The model under review builds one solid part; all positions refer to its coordinate system, in mm. Coordinates: 2 decimals unless noted, no trailing zeros. Loops run counter-clockwise (first coordinate to the right, second up) from the corner with the lowest first, then second, coordinate; pieces in that order, holes last. Notation, with made-up numbers: M -3,-35.5 L 24,-35.5 A10 cw 24,-29.5 Z; hole C -21,66.5 d2. An arc over 180 degrees is marked long. Return JSON: item names as keys, results as strings.
```python
from build123d import *

# Parameters (mm, degrees)
SKETCH1_R           = 12
SKETCH1_R_2         = 8
BOSS_EXTRUDE1_DEPTH = 10
CHAMFER1_SIZE       = 1
SKETCH2_R           = 2
CUT_EXTRUDE1_DEPTH  = 27


with BuildPart() as part:
    # Sketch1 → Boss-Extrude1 (new body)
    with BuildSketch(Plane.XY):
        Circle(SKETCH1_R)
        Circle(SKETCH1_R_2, mode=Mode.SUBTRACT)
    extrude(amount=BOSS_EXTRUDE1_DEPTH)

    # Chamfer1
    chamfer1_edges = [part.edges().sort_by_distance(p)[0] for p in [
        (-12, 0, 10),
    ]]
    chamfer(chamfer1_edges, length=CHAMFER1_SIZE)

    # Sketch2 → Cut-Extrude1 (cut, symmetric)
    with BuildSketch(Plane(origin=(0, 0, 0), x_dir=(1, 0, 0), z_dir=(0, 1, 0))):
        with Locations(Location((0, -4.2, 0), (0, 0, 270))):
            Circle(SKETCH2_R)
    extrude(amount=CUT_EXTRUDE1_DEPTH, both=True, mode=Mode.SUBTRACT)


solid = part.part
```
1. Add section B-B on y = 0. Give the boundary of the cut face in (x, z), plus the area to 3 significant figures.
Check values:
{"outline": "M -12,0 L -8,0 L -8,10 L -11,10 L -12,9 Z; M 8,0 L 12,0 L 12,9 L 11,10 L 8,10 Z", "area": "79.0 mm²"}
2. Add section A-A on x = 0. Give the boundary of the cut face in (y, z).
Check values:
{"outline": "M -12,0 L -8,0 L -8,2.2 L -12,2.2 Z; M -12,6.2 L -8,6.2 L -8,10 L -11,10 L -12,9 Z; M 8,0 L 12,0 L 12,2.2 L 8,2.2 Z; M 8,6.2 L 12,6.2 L 12,9 L 11,10 L 8,10 Z"}
3. To check wall thickness, follow line 1 (Z direction, x = 0, y = -9.2); line 2 (X direction, y = 9.15, z = 4.2); line 3 (Y direction, x = 6.5, z = 7.5). State the ranges of each line that lie inside material, in increasing order.
Check values:
{"line 1": "0 to 2.2, 6.2 to 10", "line 2": "-7.76 to -2, 2 to 7.76", "line 3": "-10.09 to -4.66, 4.66 to 10.09"}
4. Add section D-D on z = 3.5. Give the boundary of the cut face in (x, y), plus the area to 3 significant figures.
Check values:
{"outline": "M -1.87,-11.85 L -1.87,-7.78 A8 cw -1.87,7.78 L -1.87,11.85 A12 ccw Z; M 1.87,-11.85 A12 ccw 1.87,11.85 L 1.87,7.78 A8 cw 1.87,-7.78 Z", "area": "221 mm²"}
5. The part is to be moulded in two halves that separate along Z. For faces 1 (the face through (0.088, -9.845, 2.202)), 2 (the face through (-2, -8, 10)), 3 (the face through (2, -8, 0)), say which applies: released by +Z, released by -Z, zero draft, split by the parting line, or undercut.
Check values:
{"face 1": "undercut", "face 2": "released by +Z", "face 3": "released by -Z"}
6. Insertion check: pin 1 Ø6 at (y, z) = (7, 3.5) entering from -X; pin 2 Ø2 at (y, z) = (5.5, 7) entering from +X; pin 3 Ø4 at (y, z) = (-6.5, 6) entering from -X. Each pin has a flat end and moves straight along its axis. Give the tip position at first contact, or say it passes through.
Check values:
{"pin 1": "x = -11.31", "pin 2": "x = 11.12", "pin 3": "x = -11.12"}
7. Add section C-C on z = 8. Give the boundary of the cut face in (x, y).
Check values:
{"outline": "C 0,0 d24; hole C 0,0 d16"}
